CAD build for the part. Positions are in the model's coordinates, mm. Round coordinates to 2 decimals unless told otherwise and drop trailing zeros. Order: outer loops, then holes, each group sorted by start corner. A loop starts at its lowest first (then second) coordinate and runs counter-clockwise, first axis right, second up. Notation, with made-up numbers: M 68,81.5 L 101,81.5 A27 cw 101,101.5 Z; hole C 61,14 d1. An arc over 180 degrees is marked long. Answer as a JSON object with one key per item and string values. Group by question number.
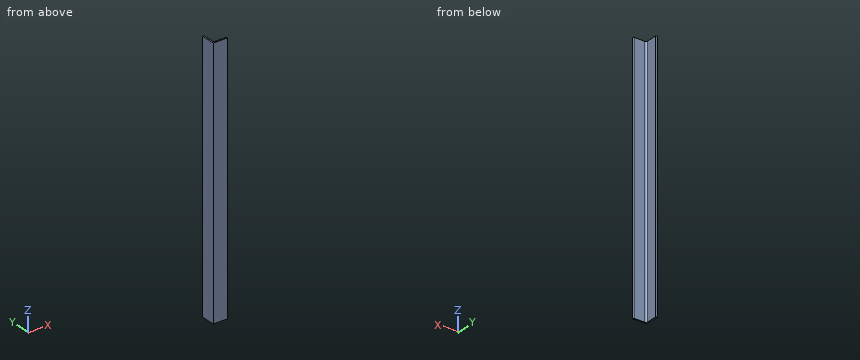
Autodesk Inventor part; units mm, degrees
ref_plane "Start plane" through (0, 0, 641.35) normal (0, 0, 1) x (1, 0, 0)
ref_plane "End plane" through (0, 0, 1797.05) normal (0, 0, 1) x (1, 0, 0)
ref_plane "YZ Plane" through (0, 0, 0) normal (1, 0, 0) x (0, 1, 0)
ref_plane "Start plane" through (0, 0, 641.35) normal (0, 0, 1) x (1, 0, 0)
ref_plane "End plane" through (0, 0, 1797.05) normal (0, 0, 1) x (1, 0, 0)
sketch "Sketch" plane through (0, 0, 0) normal (0, 0, 1) x (1, 0, 0)
  line L0 (63.5, 0) -> (0, 0)
  line L1 (0, 0) -> (0, 63.5)
  line L2 (0, 63.5) -> (2.54, 63.5)
  line L3 (6.35, 59.69) -> (6.35, 14.224)
  line L4 (14.224, 6.35) -> (59.69, 6.35)
  line L5 (63.5, 2.54) -> (63.5, 0)
  line L6 (0, -11.0414) -> (0, 31.5385) construction
  line L7 (-11.0414, 0) -> (31.5385, 0) construction
  arc A0 (6.35, 14.224) -> (14.224, 6.35) centre (14.224, 14.224) ccw
  arc A1 (6.35, 59.69) -> (2.54, 63.5) centre (2.54, 59.69) ccw
  arc A2 (63.5, 2.54) -> (59.69, 6.35) centre (59.69, 2.54) ccw
  line L8 (0, 79.3552) -> (0, -26.1075) construction
  line L9 (-26.1075, 0) -> (79.3552, 0) construction
  point P0 (6.35, 63.5)
  point P1 (6.35, 6.35)
  point P2 (63.5, 6.35)
  dimension "d0" = 63.5
  dimension "d1" = 63.5
  dimension "d2" = 6.35
  dimension "d3" = 6.35
  dimension "d10" = 0
  dimension "d11" = 0
  dimension "d14" = 7.874
  dimension "d15" = 3.81
extrude "Body" add sketch "Sketch" along normal up to surface (1155.7 mm away) from surface at 641.35
sketch "Sketch3" plane through (0, 0, 0) normal (0, 0, 1) x (1, 0, 0)
  line L0 (0, 0) -> (10, 0)
ref_plane "Work Plane3" through (0, 0, 0) normal (0, -1, 0) x (1, 0, 0)
sketch "Sketch4" plane through (0, 0, 0) normal (0, -1, 0) x (1, 0, 0)
  line L0 (-2, 641.35) -> (12, 641.35)
  line L1 (-2, 1797.05) -> (12, 1797.05)
  dimension "d17" = 1155.7
equation "\"d0\" = G_H"
equation "\"d1\" = G_H"
equation "\"d2\" = G_T"
equation "\"d3\" = G_T"
equation "\"d14\" = G_IR"
equation "\"d15\" = G_ER"
equation "\"d4\" = G_L"
equation "\"G_H\" = 63.5"
equation "\"G_T\" = 6.35"
equation "\"G_ER\" = 3.81"
equation "\"G_IR\" = 7.874"
equation "\"G_L\" = d17"
equation "\"ex\" = 0"
equation "\"G_OFFSET_START\" = -641.35"
equation "\"G_OFFSET_END\" = -641.35"
equation "\"d12\" = -G_OFFSET_START"
equation "\"d13\" = G_OFFSET_END + B_L"
equation "\"B_L\" = 2438.4"
properties part number "AISC - L 2.5 x 2.5 x 1/4 - 45.5" material "Steel, Mild"
Item 1: Cut at A-A, the plane z = 1092. Give the cut face in (x, y).
Item 2: Flat gauge pins, fed straight in: pin 1 Ø22.5 at (x, z) = (41, 1153.5) entering from +Y; pin 2 Ø1 at (y, z) = (9, 1344.5) entering from +X. Where does each tip first touch, or does it go through?
Item 3: Drill centre lines: line 1 (Y direction, x = 31.5, z = 1118); line 2 (Y direction, x = 3.5, z = 871). Where is each one in solid material? Low to high. Write a range as [from, to].
Item 4: Cut at B-B, the plane x = 47.5. Give the cut face in (y, z), and give its area (3 significant figures).
Response values:
{
 "1": {"outline": "M 0,0 L 63.5,0 L 63.5,2.54 A3.81 ccw 59.69,6.35 L 14.22,6.35 A7.87 cw 6.35,14.22 L 6.35,59.69 A3.81 ccw 2.54,63.5 L 0,63.5 Z"},
 "2": {"pin 1": "y = 6.35", "pin 2": "x = 8.82"},
 "3": {"line 1": "[0, 6.35]", "line 2": "[0, 63.38]"},
 "4": {"outline": "M 0,641.35 L 6.35,641.35 L 6.35,1797.05 L 0,1797.05 Z", "area": "7,340 mm^2"}
}
